Verification items for the finished model (mm, model axes). A direction names the side the tool comes from. Give positions to 0.01 mm unless a question says otherwise; leave off trailing zeros. Loops run counter-clockwise (first coordinate to the right, second up) from the corner with the lowest first, then second, coordinate; pieces in that order, holes last. Notation, with made-up numbers: M 0.5,19 L 40.5,19 A23 ccw 40.5,36 Z; hole C 21,-2 d10. An arc over 180 degrees is marked long. Use a Markdown table: item, result.
from build123d import *

# Parameters (mm, degrees)
SKETCH_1_R      = 1.65
EXTRUDE_1_DEPTH = 3


with BuildPart() as part:
    # 草图1 → 凸台-拉伸1 (new body)
    with BuildSketch(Plane.XY):
        with BuildLine():
            Line((-110, 25), (110, 25))
            ThreePointArc((110, 25), (117.071067812, 27.928932188), (120, 35))
            Line((120, 35), (120, 45))
            Line((120, 45), (140, 45))
            Line((140, 45), (140, -45))
            Line((140, -45), (120, -45))
            Line((120, -45), (120, -35))
            ThreePointArc((120, -35), (117.071067812, -27.928932188), (110, -25))
            Line((110, -25), (-110, -25))
            ThreePointArc((-110, -25), (-117.071067812, -27.928932188), (-120, -35))
            Line((-120, -35), (-120, -45))
            Line((-120, -45), (-140, -45))
            Line((-140, -45), (-140, 45))
            Line((-140, 45), (-120, 45))
            Line((-120, 45), (-120, 35))
            ThreePointArc((-120, 35), (-117.071067812, 27.928932188), (-110, 25))
        make_face()
        with Locations((-130, 25)):
            Circle(SKETCH_1_R, mode=Mode.SUBTRACT)
        with Locations((-130, 5)):
            Circle(SKETCH_1_R, mode=Mode.SUBTRACT)
        with Locations((-130, -15)):
            Circle(SKETCH_1_R, mode=Mode.SUBTRACT)
        with Locations((-130, -35)):
            Circle(SKETCH_1_R, mode=Mode.SUBTRACT)
        with Locations(Location((130, -35, 0), (0, 0, 180))):
            Circle(SKETCH_1_R, mode=Mode.SUBTRACT)
        with Locations(Location((130, -15, 0), (0, 0, 180))):
            Circle(SKETCH_1_R, mode=Mode.SUBTRACT)
        with Locations(Location((130, 5, 0), (0, 0, 180))):
            Circle(SKETCH_1_R, mode=Mode.SUBTRACT)
        with Locations(Location((130, 25, 0), (0, 0, 180))):
            Circle(SKETCH_1_R, mode=Mode.SUBTRACT)
    extrude(amount=EXTRUDE_1_DEPTH)


solid = part.part
(1) Material ranges on line 1 (X direction, y = 4.5, z = 2.6); line 2 (X direction, y = 4, z = 1.15); line 3 (Y direction, x = 23, z = 1.8), recorded low to high.
Results below:
| item | result |
|---|---|
| line 1 | -140 to -131.57, -128.43 to 128.43, 131.57 to 140 |
| line 2 | -140 to -131.31, -128.69 to 128.69, 131.31 to 140 |
| line 3 | -25 to 25 |
(2) Draft check along X on faces 4 (the flat face through (2, 1, 3)), 5 (the cylindrical face through (117.15, -28.01, 1.48)). Enter one of: +X half, -X half, draft (parallel to the pull), parting line (faces both ways), or undercut.
Results below:
| item | result |
|---|---|
| face 4 | draft |
| face 5 | undercut |
(3) Cross-section at B-B on x = 72.5. Record the cut outline in (y, z).
Results below:
| item | result |
|---|---|
| outline | M -25,0 L 25,0 L 25,3 L -25,3 Z |
(4) Cross-section at A-A on z = 2.25. State how many separate pieces and enclosed holes the cut face has, then the cut area to 3 significant figures.
Results below:
| item | result |
|---|---|
| separate pieces | 1 |
| enclosed holes | 8 |
| area | 15,600 mm^2 |
(5) Gauge pin test, flat ends, axial feed: P1, Ø1.5, axis at x = -6, z = 2, coming from the -Y side; P2, Ø2, axis at x = -130, y = 25, coming from the +Z side. Record the tip position at first contact, or that the pin passes through.
Results below:
| item | result |
|---|---|
| P1 | y = -25 |
| P2 | through |
(6) Set-up check for faces 1 (the cylindrical face through (116.99, 27.85, 1.48)), 2 (the cylindrical face through (-116.99, -27.85, 1.48)), 3 (the flat face through (2, 1, 0)): record each of +Z, -Z, +X, -X, +Y, -Y from which the full face is reachable in a straight line by a thin tool's end or side.
Results below:
| item | result |
|---|---|
| face 1 | +Z, -Z, +Y |
| face 2 | +Z, -Z, -Y |
| face 3 | -Z, +X, -X, +Y, -Y |
